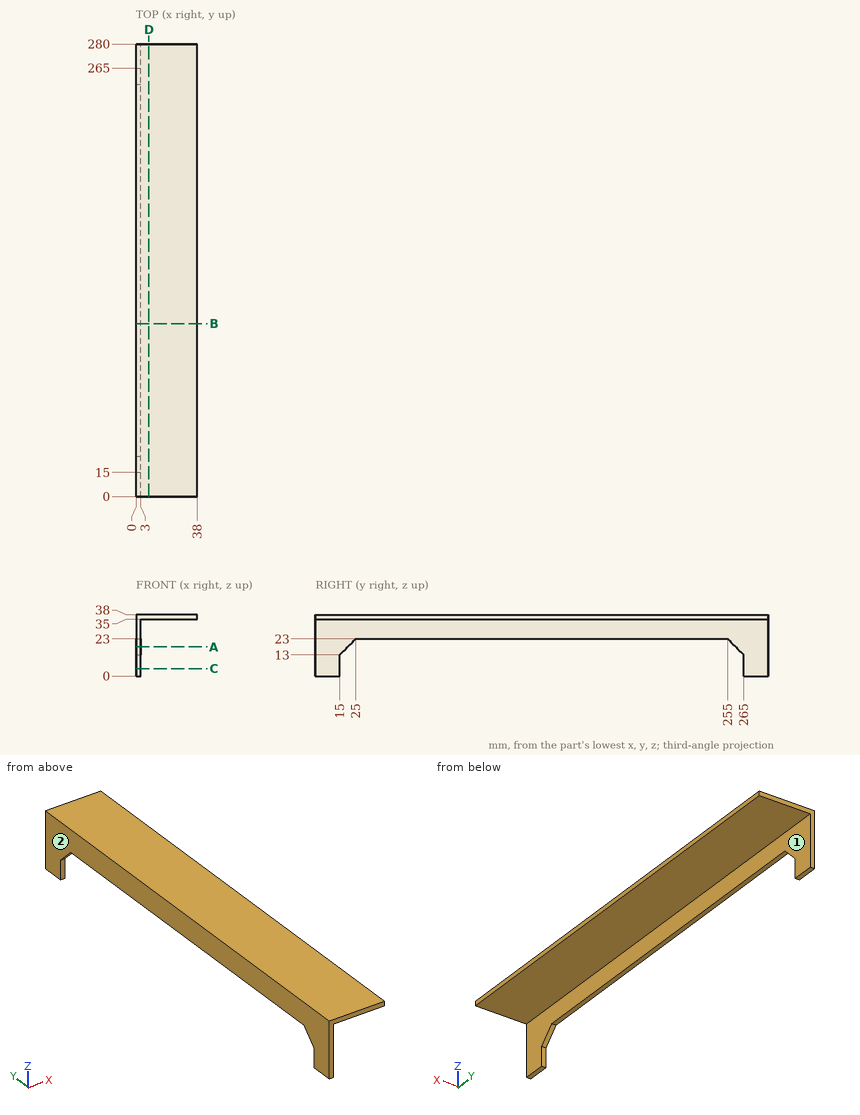
Job drawing, mm, ordinate dimensions from the low corner. One solid piece. A direction names the side the tool comes from. Give positions to 0.01 mm unless a question says otherwise; leave off trailing zeros. Order: outer loops, then holes, each group sorted by start corner. A loop starts at its lowest first (then second) coordinate and runs counter-clockwise, first axis right, second up. Notation, with made-up numbers: (18, 65) - (76, 65) arc R27 cw to (76, 81) - close; hole circle Ø9 at (37.5, 26.5). An arc over 180 degrees is marked (long way). Answer in a Markdown table with one row per item.
1. Saw through at D-D, the plane x = 8. Give the cut face in (y, z), plus the area to 3 significant figures.
Data:
| item | result |
|---|---|
| outline | (0, 35) - (280, 35) - (280, 38) - (0, 38) - close |
| area | 840 mm² |
2. Probe probe 1 along Z at (x, y) = (11, 217); probe 2 along X at (y, z) = (179, 29). List the from-to ranges inside material, lowest first. Write a range as [from, to].
Data:
| item | result |
|---|---|
| probe 1 | z = [35, 38] |
| probe 2 | x = [0, 3] |
3. Flat gauge pins, fed straight in: pin 1 (8 mm diameter, centred on x = 5.5, z = 6, fed in from -Y); pin 2 (3.5 mm diameter, centred on x = 1, y = 157, fed in from -Z); pin 3 (17.5 mm diameter, centred on x = 21, y = 202, fed in from -Z). Where does each tip first touch, or does it go through?
Data:
| item | result |
|---|---|
| pin 1 | stops at y = 0 |
| pin 2 | stops at z = 23 |
| pin 3 | stops at z = 35 |
4. Saw through at C-C, the plane z = 4.5. Give the cut face in (x, y).
Data:
| item | result |
|---|---|
| outline | (0, 0) - (3, 0) - (3, 15) - (0, 15) - close; (0, 265) - (3, 265) - (3, 280) - (0, 280) - close |
5. Saw through at B-B, the plane y = 107. Give the cut face in (x, z), plus the area to 3 significant figures.
Data:
| item | result |
|---|---|
| outline | (0, 23) - (3, 23) - (3, 35) - (38, 35) - (38, 38) - (0, 38) - close |
| area | 150 mm² |
6. Tool access for the marked faces 1 and 2: list every direction of +Z, -Z, +X, -X, +Y, -Y with a clear straight run to the whole face (end or side of a thin tool).
Data:
| item | result |
|---|---|
| face 1 | -Z, +X, +Y, -Y |
| face 2 | +Z, -Z, -X, +Y, -Y |
7. Saw through at A-A, the plane z = 18. Give the cut face in (x, y).
Data:
| item | result |
|---|---|
| outline | (0, 0) - (3, 0) - (3, 20) - (0, 20) - close; (0, 260) - (3, 260) - (3, 280) - (0, 280) - close |
